from build123d import *

# Parameters (mm, degrees)
SKETCH1_R           = 5
BOSS_EXTRUDE1_DEPTH = 2.5
SCALE1_SCALE        = 0.3


with BuildPart() as part:
    # Sketch1 → Boss-Extrude1 (new body, symmetric)
    with BuildSketch(Plane.XY):
        with BuildLine():
            Line((72.497051665, 56.504761557), (72.497051665, 11.504761557))
            ThreePointArc((72.497051665, 11.504761557), (64.997051665, 4.004761557), (57.497051665, 11.504761557))
            Line((57.497051665, 11.504761557), (57.497051665, 56.504761557))
            ThreePointArc((57.497051665, 56.504761557), (64.997051665, 64.004761557), (72.497051665, 56.504761557))
        make_face()
        with Locations((64.997051665, 56.504761557)):
            Circle(SKETCH1_R, mode=Mode.SUBTRACT)
        with Locations((64.997051665, 11.504761557)):
            Circle(SKETCH1_R, mode=Mode.SUBTRACT)
    extrude(amount=BOSS_EXTRUDE1_DEPTH, both=True)


with BuildPart() as part_1:
    # Scale1: scaled about (64.997051665, 34.004761557, 0)
    add(part.part.scale(SCALE1_SCALE).moved(Location((45.497936166, 23.80333309, 0))))


solid = part_1.part
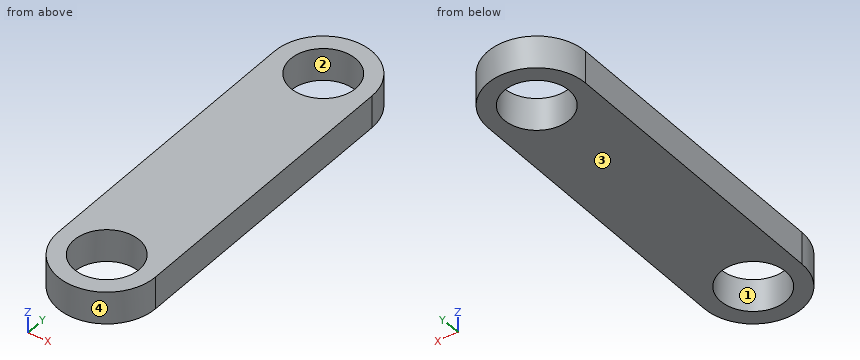
Design review of the part built by this model. Coordinates are the model's own, in mm. Face numbers are marked on the shaded views. Coordinates: 2 decimals unless noted, no trailing zeros. Loops run counter-clockwise (first coordinate to the right, second up) from the corner with the lowest first, then second, coordinate; pieces in that order, holes last. Notation, with made-up numbers: (-4.75, 25) -> (50.25, 25) arc R15 ccw to (50.25, 46) -> close; hole circle Ø1 at (10, 50.25). An arc over 180 degrees is marked (long way). Use a Markdown table: item, result. Add a question column.
Item 1: The part is to be moulded in two halves that separate along X. For the marked faces 1, 2, 3 and 4, say which applies: +X half, -X half, draft (parallel to the pull), parting line (faces both ways), or undercut.
Item 2: We need section B-B, the plane y = 27. Write out the cut boundary in (x, z), and give its area (3 significant figures).
Item 3: We need section A-A, the plane x = 65. Write out the cut boundary in (y, z).
Item 4: We need section D-D, the plane x = 66.2. Write out the cut boundary in (y, z), and give its area (3 significant figures).
Item 5: Wall thickness on L1, parallel to Y at x = 65.1, z = 0.45; L2, parallel to Y at x = 65.9, z = -0.35; L3, parallel to X at y = 40.75, z = 0.45: over which ranges is each line inside the solid? List them lowest first. Write a range as from..to.
Item 6: We need section C-C, the plane z = 0.45. Write out the cut boundary in (x, y), and give its area (3 significant figures).
Numbers:
| question | item | result |
|---|---|---|
| 1 | face 1 | undercut |
| 1 | face 2 | undercut |
| 1 | face 3 | draft |
| 1 | face 4 | parting line |
| 2 | outline | (62.76, -0.75) -> (63.52, -0.75) -> (63.52, 0.75) -> (62.76, 0.75) -> close; (66.48, -0.75) -> (67.23, -0.75) -> (67.23, 0.75) -> (66.48, 0.75) -> close |
| 2 | area | 2.27 mm^2 |
| 3 | outline | (25, -0.75) -> (25.75, -0.75) -> (25.75, 0.75) -> (25, 0.75) -> close; (28.75, -0.75) -> (39.25, -0.75) -> (39.25, 0.75) -> (28.75, 0.75) -> close; (42.25, -0.75) -> (43, -0.75) -> (43, 0.75) -> (42.25, 0.75) -> close |
| 4 | outline | (25.35, -0.75) -> (26.36, -0.75) -> (26.36, 0.75) -> (25.35, 0.75) -> close; (28.15, -0.75) -> (39.86, -0.75) -> (39.86, 0.75) -> (28.15, 0.75) -> close; (41.65, -0.75) -> (42.66, -0.75) -> (42.66, 0.75) -> (41.65, 0.75) -> close |
| 4 | area | 20.6 mm^2 |
| 5 | L1 | y = 25.01..25.76, 28.75..39.26, 42.25..43 |
| 5 | L2 | y = 25.19..26.06, 28.45..39.56, 41.95..42.82 |
| 5 | L3 | x = 62.75..63.5, 66.5..67.25 |
| 6 | outline | (62.75, 27.25) arc R2.25 ccw to (67.25, 27.25) -> (67.25, 40.75) arc R2.25 ccw to (62.75, 40.75) -> close; hole circle Ø3 at (65, 27.25); hole circle Ø3 at (65, 40.75) |
| 6 | area | 62.5 mm^2 |
